Input: part model. Units: mm. Frame: model coordinates. Face numbers are marked on the shaded views. Round coordinates to 2 decimals unless told otherwise and drop trailing zeros. Order: outer loops, then holes, each group sorted by start corner. A loop starts at its lowest first (then second) coordinate and runs counter-clockwise, first axis right, second up. Notation, with made-up numbers: (44.5, -9) - (60.5, -9) arc R20 ccw to (60.5, 6) - close; hole circle Ø9 at (21, 47.25). An arc over 180 degrees is marked (long way). One line per item, written item: value. Start each with the question number.
from build123d import *

# Parameters (mm, degrees)
ESBO_O1_W                                  = 22
ESBO_O1_H                                  = 12
RESSALTO_EXTRUS_O1_DEPTH                   = 5
BROCA_DE_ROSQUEAR_PARA_TARRAXA_DE_M8X1_0_D = 7
BROCA_DE_ROSQUEAR_PARA_TARRAXA_DE_M4X0_7_D = 3.3
FILETE1_R                                  = 1


with BuildPart() as part:
    # Esboço1 → Ressalto-extrusão1 (new body)
    with BuildSketch(Plane.XY):
        with Locations((-43.64943678, -9.559141583)):
            Rectangle(ESBO_O1_W, ESBO_O1_H)
    extrude(amount=RESSALTO_EXTRUS_O1_DEPTH)

    # Broca de rosquear para tarraxa de M8x1.01 (through all)
    with Locations(Plane.XY.offset(5)):
        with Locations((-38.64943678, -9.559141583)):
            Hole(BROCA_DE_ROSQUEAR_PARA_TARRAXA_DE_M8X1_0_D / 2)

    # Broca de rosquear para tarraxa de M4x0.71 (through all)
    with Locations(Plane.XY.offset(5)):
        with Locations((-50.64943678, -9.559141583)):
            Hole(BROCA_DE_ROSQUEAR_PARA_TARRAXA_DE_M4X0_7_D / 2)

    # Filete1
    filete1_edges = [part.edges().sort_by_distance(p)[0] for p in [
        (-35.14943678, -9.559141583, 5),
    ]]
    fillet(filete1_edges, radius=FILETE1_R)


solid = part.part
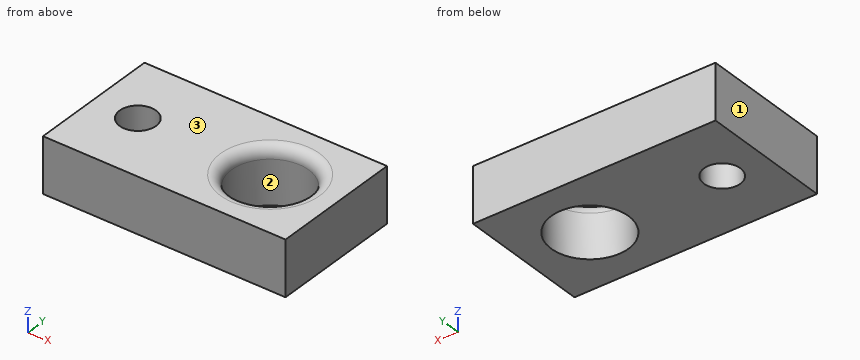
Item 1: Line query: L1, parallel to X at y = -10.75, z = 1.7; L2, parallel to X at y = -9.25, z = 3.7; L3, parallel to Y at x = -41, z = 2.1. Output: solid intervals per line, ascending.
Item 2: Section query C-C on z = 4.35. Return loops of the section in (x, y), and give its area (3 significant figures).
Item 3: Section query A-A on z = 2.6. Return loops of the section in (x, y), and give its area (3 significant figures).
Item 4: Section query B-B on y = -10.25. Give the number of separate pieces and of enclosed holes in the cut face, and give its area (3 significant figures).
Item 5: Pull-direction query (X, two-part tool) for the marked faces 1, 2 and 3; classes: released by +X, released by -X, zero draft, split by the parting line, or undercut.
Geometry results:
1. L1: x = -54.65 to -51.79, -49.51 to -41.94, -35.36 to -32.65
1. L2: x = -54.65 to -52.27, -49.03 to -42.14, -35.16 to -32.65
1. L3: y = -15.56 to -12.15, -6.97 to -3.56
2. outline: (-54.65, -15.56) - (-32.65, -15.56) - (-32.65, -3.56) - (-54.65, -3.56) - close; hole circle Ø3.3 at (-50.65, -9.56); hole circle Ø7.13 at (-38.65, -9.56)
2. area: 216 mm^2
3. outline: (-54.65, -15.56) - (-32.65, -15.56) - (-32.65, -3.56) - (-54.65, -3.56) - close; hole circle Ø3.3 at (-50.65, -9.56); hole circle Ø7 at (-38.65, -9.56)
3. area: 217 mm^2
4. separate pieces: 3
4. enclosed holes: 0
4. area: 60.3 mm^2
5. face 1: released by -X
5. face 2: undercut
5. face 3: zero draft
